```python
from build123d import *

# Parameters (mm, degrees)
CIRPATTERN1_COUNT = 3


with BuildPart() as part:
    # Sketch1 → Revolve1 (revolve)
    with BuildSketch(Plane.XY):
        Polygon((0, 14.478), (41.148, 14.478), (41.148, 15.9385), (48.895, 15.9385), (48.895, 15.237243561), (24.638, 8.7376), (24.638, 10.3251), (7.62, 10.3251), (7.62, 11.1633), (5.842, 11.1633), (5.842, 12.7), (0, 12.7), align=None)
    revolve(axis=Axis((0, 0, 0), (1, 0, 0)))

    # Sketch3 → #6-32 Tapped Hole1 (revolve, cut)
    with BuildSketch(Plane(origin=(28.448, 14.478, 0), x_dir=(0, 0, 1), z_dir=(1, 0, 0))):
        Polygon((0, 0), (0, 3.175), (1.35255, 2.36230597), (1.35255, 0), align=None)
    f_6_32_tapped_hole1 = revolve(axis=Axis((28.448, 20.828, 0), (0, -1, 0)), mode=Mode.SUBTRACT)

    # CirPattern1: #6-32 Tapped Hole1 ×3 about axis
    cirpattern1_axis = Axis((0, 0, 0), (-1, 0, 0))
    for i in range(1, CIRPATTERN1_COUNT):
        add(f_6_32_tapped_hole1.rotate(cirpattern1_axis, i * 360 / CIRPATTERN1_COUNT), mode=Mode.SUBTRACT)


solid = part.part
```
CAD build for the part. Positions are in the model's coordinates, mm. A direction names the side the tool comes from. Coordinates: 2 decimals unless noted, no trailing zeros. Order: outer loops, then holes, each group sorted by start corner. A loop starts at its lowest first (then second) coordinate and runs counter-clockwise, first axis right, second up. Notation, with made-up numbers: M -36.75,1.25 L 8.25,1.25 A18 cw 8.25,27.25 Z; hole C -36,55 d4. An arc over 180 degrees is marked long. Write each question's results on one line, items separated by ' | '. Start each with the question number.
Q1. Which spindle directions (+Z, -Z, +X, -X, +Y, -Y) get a long thin tool onto all of the face, cutting with end or side? Do faces 4 (the conical face through (33.9, 10.7, 3.37)), 5 (the flat face through (7.62, -7, -8)), 6 (the cylindrical face through (27.107, 13.313, -0.176)), 7 (the conical face through (28.215, -5.696, 9.926)). Say none if no direction does.
Q2. Drill centre lines: probe 1 along Z at (x, y) = (16, 0); probe 2 along Z at (x, y) = (3.3, 0); probe 3 along Y at (x, z) = (13, 5.5). Where is each one in solid material? Low to high. Write a range as from..to.
Q3. Flat gauge pins, fed straight in: P1, Ø6, axis at x = 8.5, y = -1.5, coming from the +Z side; P2, Ø4, axis at x = 29, y = 3, coming from the -Z side; P3, Ø2, axis at x = 35, z = -12, coming from the -Y side. Where does each tip first touch, or does it go through?
Q4. Cut at C-C (x = 39). List the corners of the cut face in (y, z), then the cut area to 3 significant figures.
Q5. Pull direction Y, two halves, no side cores. Call faces 1 (the conical face through (28.215, -5.749, -9.896)), 2 (the cylindrical face through (20.862, -1.885, 14.355)), 3 (the flat face through (0, 0, -13)): +Y half, -Y half, draft (parallel to the pull), parting line (faces both ways), or undercut.
Q6. Cut at B-B (x = 11). List the corners of the cut face in (y, z).
Q7. Cut at A-A (y = 0). List the corners of the cut face in (x, z) (1 decimal).
Found:
1) face 4: +X | face 5: -X | face 6: +Y | face 7: none
2) probe 1: -14.48..-10.33, 10.33..14.48 | probe 2: -14.48..-12.7, 12.7..14.48 | probe 3: -13.39..-8.74, 8.74..13.39
3) P1: z = 14.48 | P2: z = -14.44 | P3: y = -9.41
4) outline: C 0,0 d28.96; hole C 0,0 d25.17 | area: 161 mm²
5) face 1: undercut | face 2: parting line | face 3: draft
6) outline: C 0,0 d28.96; hole C 0,0 d20.65
7) outline: M 0,-14.5 L 41.1,-14.5 L 41.1,-15.9 L 48.9,-15.9 L 48.9,-15.2 L 24.6,-8.7 L 24.6,-10.3 L 7.6,-10.3 L 7.6,-11.2 L 5.8,-11.2 L 5.8,-12.7 L 0,-12.7 Z; M 0,12.7 L 5.8,12.7 L 5.8,11.2 L 7.6,11.2 L 7.6,10.3 L 24.6,10.3 L 24.6,8.7 L 48.9,15.2 L 48.9,15.9 L 41.1,15.9 L 41.1,14.5 L 0,14.5 Z
